Build history of the part. All positions in model axes, mm. A direction names the side the tool comes from. Round coordinates to 2 decimals unless told otherwise and drop trailing zeros. Loops run counter-clockwise (first coordinate to the right, second up) from the corner with the lowest first, then second, coordinate; pieces in that order, holes last.
Autodesk Inventor part; units mm, degrees
ref_plane "YZ Plane" through (0, 0, 0) normal (1, 0, 0) x (0, 1, 0)
ref_plane "XZ Plane" through (0, 0, 0) normal (0, 1, 0) x (-1, 0, 0)
ref_plane "XY Plane" through (0, 0, 0) normal (0, 0, 1) x (1, 0, 0)
sketch "Sketch1" plane through (0, 0, 0) normal (0, 0, 1) x (1, 0, 0)
  circle A0 centre (0, 0) radius 7.62
  line L0 (-7.62, 0) -> (-7.62, 5.08)
  line L1 (0, -7.62) -> (-5.08, -7.62)
  line L2 (0, -7.62) -> (5.08, -7.62)
  line L3 (-7.62, 0) -> (-5.08, -7.62)
  line L4 (5.08, -7.62) -> (7.62, 0)
  line L5 (7.62, 0) -> (7.62, 5.08)
  line L6 (-7.62, 5.08) -> (-10.16, 5.08)
  line L7 (-10.16, 5.08) -> (-10.16, 0)
  line L8 (-5.08, -7.62) -> (-6.7733, -10.16)
  line L9 (-6.7733, -10.16) -> (-10.16, 0)
  line L10 (7.62, 5.08) -> (10.16, 5.08)
  line L11 (10.16, 5.08) -> (10.16, 0)
  line L12 (10.16, 0) -> (6.7733, -10.16)
  line L13 (6.7733, -10.16) -> (-6.7733, -10.16)
  line L14 (5.08, -7.62) -> (6.7733, -10.16)
  dimension "d0" = 15.24
  dimension "d1" = 5.08
  dimension "d2" = 5.08
  dimension "d3" = 5.08
  dimension "d4" = 5.08
  dimension "d6" = 2.54
  dimension "d7" = 2.54
  dimension "d8" = 2.54
extrude "Extrusion1" add sketch "Sketch1" along normal blind 152.4 contours L5 L10 L11 L12 L14 L4 A0 | A0 L4 | L3 A0 | A0 L3 L8 L9 L7 L6 L0 | L2 L14 L13 L8 L1
properties part number "StraightTrackv2"
(1) Probe line 1 (X direction, y = 0.75, z = 23.5); line 2 (X direction, y = -7.5, z = 135); line 3 (Y direction, x = 0.5, z = 41). List the from-to ranges inside material, lowest first.
Responses:
line 1: x = -10.16 to -7.62, 7.62 to 10.16
line 2: x = -7.66 to -5.12, 5.12 to 7.66
line 3: y = -10.16 to -7.62
(2) Pull direction X, two halves, no side cores. Call faces 1 (the face through (-8.443, -5.151, 75.133)), 2 (the face through (10.16, 3, 75)), 3 (the face through (0, -7.62, 75)), 4 (the face through (0, -10.16, 75)): +X half, -X half, draft (parallel to the pull), parting line (faces both ways), or undercut.
Responses:
face 1: -X half
face 2: +X half
face 3: undercut
face 4: draft
(3) Slice it at C-C on x = -1.75. List the corners of the cut face in (y, z), plus the area to 3 significant figures.
Responses:
outline: (-10.16, 0) - (-7.62, 0) - (-7.62, 152.4) - (-10.16, 152.4) - close
area: 387 mm2
(4) Slice it at D-D on y = -3.75. List the corners of the cut face in (x, z).
Responses:
outline: (-8.91, 0) - (-6.37, 0) - (-6.37, 152.4) - (-8.91, 152.4) - close; (6.37, 0) - (8.91, 0) - (8.91, 152.4) - (6.37, 152.4) - close
(5) Slice it at B-B on z = 139. List the corners of the cut face in (x, y).
Responses:
outline: (-10.16, 0) - (-6.77, -10.16) - (6.77, -10.16) - (10.16, 0) - (10.16, 5.08) - (7.62, 5.08) - (7.62, 0) - (5.08, -7.62) - (-5.08, -7.62) - (-7.62, 0) - (-7.62, 5.08) - (-10.16, 5.08) - close
(6) Which spindle directions (+Z, -Z, +X, -X, +Y, -Y) get a long thin tool onto all of the face, cutting with end or side? Do faces 5 (the face through (-7.62, 3, 75)), 6 (the face through (9, 5.08, 75)). Say none if no direction does.
Responses:
face 5: +Z, -Z, +Y
face 6: +Z, -Z, +X, -X, +Y
(7) Slice it at A-A on y = 2. List the corners of the cut face in (x, z), plus the area to 3 significant figures.
Responses:
outline: (-10.16, 0) - (-7.62, 0) - (-7.62, 152.4) - (-10.16, 152.4) - close; (7.62, 0) - (10.16, 0) - (10.16, 152.4) - (7.62, 152.4) - close
area: 774 mm2
(8) Pin check, flat tips, straight feed: P1, Ø1.5, axis at x = 0.5, z = 59, coming from the +Y side; P2, Ø3, axis at y = -8.5, z = 59.5, coming from the -X side. Stop position of each tip, or through.
Responses:
P1: stops at y = -7.62
P2: stops at x = -7.83
